```python
from build123d import *

# Parameters (mm, degrees)
SKETCH_1_W          = 2
SKETCH_1_H          = 1.5
CUT_EXTRUDE_1_DEPTH = 6.172040216


with BuildPart() as part:
    # Эскиз1 → Повернуть1 (revolve)
    with BuildSketch(Plane.XY, mode=Mode.PRIVATE) as revolve_1_sk:
        with Locations((2.5, 0.75)):
            Rectangle(SKETCH_1_W, SKETCH_1_H)
    revolve(revolve_1_sk.sketch.rotate(Axis((0, 0, 0), (0, 1, 0)), 90), axis=Axis((0, 0, 0), (0, 1, 0)))

    # Эскиз2 → Вырез-Вытянуть1 (cut, through all)
    with BuildSketch(Plane(origin=(0, 1.5, 0), x_dir=(1, 0, 0), z_dir=(0, 1, 0))):
        with BuildLine():
            Line((-0.7, 2), (-0.7, 3.42928564))
            ThreePointArc((-0.7, 3.42928564), (-1.923801659, 2.923865109), (-2.872281323, 2))
            Line((-2.872281323, 2), (-0.7, 2))
        make_face()
        with BuildLine():
            ThreePointArc((3.491096592, -0.249488641), (3.352391998, 1.005717599), (2.777252031, 2.129993229))
            ThreePointArc((2.777252031, 2.129993229), (1.802717143, 0.540815143), (3.491096592, -0.249488641))
        make_face()
    extrude(amount=-CUT_EXTRUDE_1_DEPTH, mode=Mode.SUBTRACT)


solid = part.part
```
Part model, mm, in its own coordinate system. A direction names the side the tool comes from. Round coordinates to 2 decimals unless told otherwise and drop trailing zeros. Write each loop counter-clockwise with the first axis right and the second up, starting at its lowest first coordinate (ties: lowest second). Pieces come first, ordered by that corner, then holes. Notation, with made-up numbers: (44.25, 23.25) -> (78.25, 23.25) arc R16 ccw to (78.25, 43.25) -> close; hole circle Ø10 at (34, -2). An arc over 180 degrees is marked (long way). Return JSON: item names as keys, results as strings. Group by question number.
Q1. Saw through at A-A on x = 0. Write the cut outline in (y, z), plus the area to 3 significant figures.
Q2. Saw through at B-B on z = -0.9. Write the cut outline in (x, y), plus the area to 3 significant figures.
Q3. Probe L1, parallel to Z at x = 2.5, y = 1.1; L2, parallel to X at y = 0.1, z = -1; L3, parallel to X at y = 0.9, z = 1.25. List the from-to ranges inside material, lowest first. Write a range as [from, to].
Q4. Which spindle directions (+Z, -Z, +X, -X, +Y, -Y) get a long thin tool onto all of the face, cutting with end or side? Do faces 1 (the flat face through (0, 0, 2)), 2 (the flat face through (-0.7, 1, -3)). Say none if no direction does.
Q5. Mould opens along Z. For faces 3 (the cylindrical face through (-1.25, 0.76, 3.27)), 4 (the flat face through (-2, 1, -2)), 5 (the cylindrical face through (1.795, 0.76, -0.569)), 6 (the flat face through (0, 1.5, 2)) say: pulls with the +Z half, pulls with the -Z half, needs draft (parallel to the pull), parting line crosses it, or undercut.
Q6. Pin check, flat tip, straight feed: pin 1 (2.5 mm diameter, centred on x = 0, z = 0, fed in from -Y). Stop position of the tip, or through.
Q7. Saw through at C-C on y = 0.35. Write the cut outline in (x, z), plus the area to 3 significant figures.
Q8. Saw through at D-D on x = -2.25. Write the cut outline in (y, z).
Answer:
{
 "1": {"outline": "(0, -3.5) -> (1.5, -3.5) -> (1.5, -1.5) -> (0, -1.5) -> close; (0, 1.5) -> (1.5, 1.5) -> (1.5, 3.5) -> (0, 3.5) -> close", "area": "6.00 mm2"},
 "2": {"outline": "(-3.38, 0) -> (-1.2, 0) -> (-1.2, 1.5) -> (-3.38, 1.5) -> close; (1.2, 0) -> (1.75, 0) -> (1.75, 1.5) -> (1.2, 1.5) -> close", "area": "4.10 mm2"},
 "3": {"L1": "[-2.45, -2.05], [0.25, 2.45]", "L2": "[-3.35, -1.12], [1.12, 1.75]", "L3": "[-3.27, -0.83], [0.83, 3.27]"},
 "4": {"face 1": "+Z, -Z, +X, -X, -Y", "face 2": "-Z, -X, +Y, -Y"},
 "5": {"face 3": "parting line crosses it", "face 4": "pulls with the -Z half", "face 5": "undercut", "face 6": "needs draft"},
 "6": {"pin 1": "through"},
 "7": {"outline": "(-2.87, -2) -> (-0.7, -2) -> (-0.7, -3.43) arc R3.5 ccw to (2.78, -2.13) arc R1.25 cw (long way) to (3.49, 0.25) arc R3.5 ccw (long way) to start; hole circle Ø3 at (0, 0)", "area": "26.2 mm2"},
 "8": {"outline": "(0, -2) -> (1.5, -2) -> (1.5, 2.68) -> (0, 2.68) -> close"}
}
